Part model, mm, in its own coordinate system. A direction names the side the tool comes from. Round coordinates to 2 decimals unless told otherwise and drop trailing zeros. Order: outer loops, then holes, each group sorted by start corner. A loop starts at its lowest first (then second) coordinate and runs counter-clockwise, first axis right, second up. Notation, with made-up numbers: (73.5, 68) -> (99.5, 68) arc R26 cw to (99.5, 106) -> close; hole circle Ø8 at (-26.75, -22.75). An arc over 180 degrees is marked (long way). Return JSON: item names as keys, results as strings. Group by question number.
from build123d import *

# Parameters (mm, degrees)
SKETCH1_R           = 4
BOSS_EXTRUDE1_DEPTH = 5
BOSS_EXTRUDE2_DEPTH = 15
SKETCH3_R           = 7.5
SKETCH3_R_2         = 4
BOSS_EXTRUDE3_DEPTH = 5
SKETCH5_R           = 4
CUT_EXTRUDE1_DEPTH  = 5
SKETCH6_R           = 7.5
BOSS_EXTRUDE4_DEPTH = 5
SKETCH7_R           = 4
CUT_EXTRUDE2_DEPTH  = 5
BOSS_EXTRUDE5_DEPTH = 15
SKETCH9_R           = 7.5
BOSS_EXTRUDE6_DEPTH = 5
SKETCH10_R          = 7.5
BOSS_EXTRUDE7_DEPTH = 5
SKETCH11_R          = 4
CUT_EXTRUDE3_DEPTH  = 64


with BuildPart() as part:
    # Sketch1 → Boss-Extrude1 (new body)
    with BuildSketch(Plane(origin=(0, 0, 0), x_dir=(0, 0, -1), z_dir=(1, 0, 0))):
        with BuildLine():
            Line((15, 0), (0, 0))
            Line((0, 0), (0, -15.59))
            ThreePointArc((0, -15.59), (1.276909506, -19.776065539), (4.672838586, -22.536737244))
            Line((4.672838586, -22.536737244), (37.484806943, -35.890449582))
            Line((37.484806943, -35.890449582), (43.13912977, -21.996975093))
            Line((43.13912977, -21.996975093), (19.672838586, -12.446737244))
            ThreePointArc((19.672838586, -12.446737244), (16.276909506, -9.686065539), (15, -5.5))
            Line((15, -5.5), (15, 0))
        make_face()
        with Locations((7.5, -16.462434129)):
            Circle(SKETCH1_R, mode=Mode.SUBTRACT)
    extrude(amount=BOSS_EXTRUDE1_DEPTH)

    # Sketch2 → Boss-Extrude2 (add)
    with BuildSketch(Plane.XY):
        with BuildLine():
            Line((0, 0), (5, 0))
            ThreePointArc((5, 0), (5.732233047, 1.767766953), (7.5, 2.5))
            ThreePointArc((7.5, 2.5), (9.267766953, 3.232233047), (10, 5))
            Line((10, 5), (10, 19.86))
            Line((10, 19.86), (5, 19.86))
            Line((5, 19.86), (5, 7.5))
            Line((5, 7.5), (0, 7.5))
            Line((0, 7.5), (0, 19.86))
            Line((0, 19.86), (-5, 19.86))
            Line((-5, 19.86), (-5, 5))
            ThreePointArc((-5, 5), (-4.267766953, 3.232233047), (-2.5, 2.5))
            ThreePointArc((-2.5, 2.5), (-0.732233047, 1.767766953), (0, 0))
        make_face()
    extrude(amount=-BOSS_EXTRUDE2_DEPTH)

    # Sketch3 → Boss-Extrude3 (add)
    with BuildSketch(Plane(origin=(10, 0, 0), x_dir=(0, 0, -1), z_dir=(1, 0, 0))):
        with Locations((7.5, 19.86)):
            Circle(SKETCH3_R)
        with Locations((7.5, 19.86)):
            Circle(SKETCH3_R_2, mode=Mode.SUBTRACT)
    extrude(amount=-BOSS_EXTRUDE3_DEPTH)

    # Sketch5 → Cut-Extrude1 (cut)
    with BuildSketch(Plane(origin=(10, 0, 0), x_dir=(0, 0, -1), z_dir=(1, 0, 0))):
        with Locations((7.5, 19.86)):
            Circle(SKETCH5_R)
    extrude(amount=-CUT_EXTRUDE1_DEPTH, mode=Mode.SUBTRACT)

    # Sketch6 → Boss-Extrude4 (add)
    with BuildSketch(Plane.ZY.offset(5)):
        with Locations((-7.5, 19.86)):
            Circle(SKETCH6_R)
    extrude(amount=-BOSS_EXTRUDE4_DEPTH)

    # Sketch7 → Cut-Extrude2 (cut)
    with BuildSketch(Plane.ZY.offset(5)):
        with Locations((-7.5, 19.86)):
            Circle(SKETCH7_R)
    extrude(amount=-CUT_EXTRUDE2_DEPTH, mode=Mode.SUBTRACT)

    # Sketch8 → Boss-Extrude5 (add)
    with BuildSketch(Plane(origin=(0, -3.809395954, 1.55033606), x_dir=(1, 0, 0), z_dir=(0, 0.926231633, -0.376954855))):
        with BuildLine():
            Line((0, 48.248693155), (5, 48.248693155))
            Line((5, 48.248693155), (24.55634321, 57.895622609))
            ThreePointArc((24.55634321, 57.895622609), (25.552769913, 58.816883816), (25.92108759, 60.122996551))
            Line((25.92108759, 60.122996551), (25.92108759, 74.712996551))
            Line((25.92108759, 74.712996551), (20.92108759, 74.712996551))
            Line((20.92108759, 74.712996551), (20.92108759, 64.128787942))
            ThreePointArc((20.92108759, 64.128787942), (20.552769913, 62.822675208), (19.55634321, 61.901414001))
            Line((19.55634321, 61.901414001), (2.258260879, 53.528693155))
            Line((2.258260879, 53.528693155), (-14.685235236, 61.886733815))
            ThreePointArc((-14.685235236, 61.886733815), (-15.702336235, 62.808740922), (-16.079254544, 64.128787942))
            Line((-16.079254544, 64.128787942), (-16.079254544, 74.791257758))
            Line((-16.079254544, 74.791257758), (-21.079254544, 74.791257758))
            Line((-21.079254544, 74.791257758), (-21.079254544, 60.201257758))
            ThreePointArc((-21.079254544, 60.201257758), (-20.702336235, 58.881210738), (-19.685235236, 57.95920363))
            Line((-19.685235236, 57.95920363), (0, 48.248693155))
        make_face()
    extrude(amount=-BOSS_EXTRUDE5_DEPTH)

    # Sketch9 → Boss-Extrude6 (add)
    with BuildSketch(Plane(origin=(25.92108759, 0, 0), x_dir=(0, 0, -1), z_dir=(1, 0, 0))):
        with Locations((64.824043295, -38.919559991)):
            Circle(SKETCH9_R)
    extrude(amount=-BOSS_EXTRUDE6_DEPTH)

    # Sketch10 → Boss-Extrude7 (add)
    with BuildSketch(Plane.ZY.offset(21.079254544)):
        with Locations((-64.896531301, -38.949060933)):
            Circle(SKETCH10_R)
    extrude(amount=-BOSS_EXTRUDE7_DEPTH)

    # Sketch11 → Cut-Extrude3 (cut)
    with BuildSketch(Plane(origin=(25.92108759, 0, 0), x_dir=(0, 0, -1), z_dir=(1, 0, 0))):
        with Locations((64.896531301, -38.949060933)):
            Circle(SKETCH11_R)
    extrude(amount=-CUT_EXTRUDE3_DEPTH, mode=Mode.SUBTRACT)


solid = part.part
(1) Tool access for faces 1 (the flat face through (2, 7, -15)), 2 (the flat face through (14.641, -30.639, -44.757)), 3 (the flat face through (-6.095, -32.39, -49.059)), 4 (the flat face through (3, 7.5, -7)): list every direction of +Z, -Z, +X, -X, +Y, -Y with a clear straight run to the whole face (end or side of a thin tool).
(2) Probe L1, parallel to X at y = 14, z = -6; L2, parallel to Z at x = 24, y = -39; L3, parallel to Z at x = 23.5, y = -37. List the from-to ranges inside material, lowest first. Write a range as [from, to].
(3) Mould opens along Y. For faces 5 (the flat face through (5, 15, -7)), 6 (the cylindrical face through (-18.614, -41.623, -71.904)), 7 (the cylindrical face through (2.46, -19.72, -1.24)), 8 (the cylindrical face through (7.535, 20.036, -3.504)) say: pulls with the +Y half, pulls with the -Y half, needs draft (parallel to the pull), parting line crosses it, or undercut.
(4) Saw through at B-B, the plane z = -7.5. List the corners of the cut face in (x, y), and give its area (3 significant figures).
(5) Saw through at A-A, the plane x = 8.5. List the corners of the cut face in (y, z).
(6) Pin check, flat tips, straight feed: P1, Ø13, axis at y = 19.86, z = -7.5, coming from the +X side; P2, Ø16.5, axis at y = 14, z = -4, coming from the -X side; P3, Ø4, axis at x = -6, z = -47, coming from the +Y side. Stop position of each tip, or through.
(7) Saw through at D-D, the plane y = 6.5. List the corners of the cut face in (x, z), and give its area (3 significant figures).
(8) Saw through at C-C, the plane z = -38.5. List the corners of the cut face in (x, y), and give its area (3 significant figures).
Results are:
{
 "1": {"face 1": "-Z, +X, -X, +Y", "face 2": "+Z, +X, +Y", "face 3": "-Z, -Y", "face 4": "+Z, -Z, +Y"},
 "2": {"L1": "x = [-5, 0], [5, 10]", "L2": "z = [-72.32, -68.9], [-60.9, -46.34]", "L3": "z = [-72.07, -68.39], [-61.4, -46.89]"},
 "3": {"face 5": "needs draft", "face 6": "parting line crosses it", "face 7": "pulls with the -Y half", "face 8": "undercut"},
 "4": {"outline": "(-5, 5) arc R2.5 ccw to (-2.5, 2.5) arc R2.5 cw to (0, 0) -> (0, -12.46) -> (5, -12.46) -> (5, 0) arc R2.5 cw to (7.5, 2.5) arc R2.5 ccw to (10, 5) -> (10, 15.86) -> (5, 15.86) -> (5, 7.5) -> (0, 7.5) -> (0, 15.86) -> (-5, 15.86) -> close; (-5, 23.86) -> (0, 23.86) -> (0, 27.36) -> (-5, 27.36) -> close; (0, -23.69) -> (5, -23.69) -> (5, -20.46) -> (0, -20.46) -> close; (5, 23.86) -> (10, 23.86) -> (10, 27.36) -> (5, 27.36) -> close", "area": "285 mm^2"},
 "5": {"outline": "(-39.02, -45.17) -> (-25.13, -50.83) -> (-22.65, -44.74) -> (-36.54, -39.08) -> close; (2.71, -15) -> (19.86, -15) arc R7.5 ccw to (19.86, 0) -> (2.71, 0) -> close; hole circle Ø8 at (19.86, -7.5)"},
 "6": {"P1": "stops at x = 10", "P2": "stops at x = -5", "P3": "stops at y = -22.9"},
 "7": {"outline": "(-5, -15) -> (10, -15) -> (10, 0) -> (-5, 0) -> close", "area": "225 mm^2"},
 "8": {"outline": "(-2.22, -36.3) -> (7.22, -36.3) -> (5, -33.4) -> (5, -20.11) -> (0, -20.11) -> (0, -33.4) -> close", "area": "87.4 mm^2"}
}
